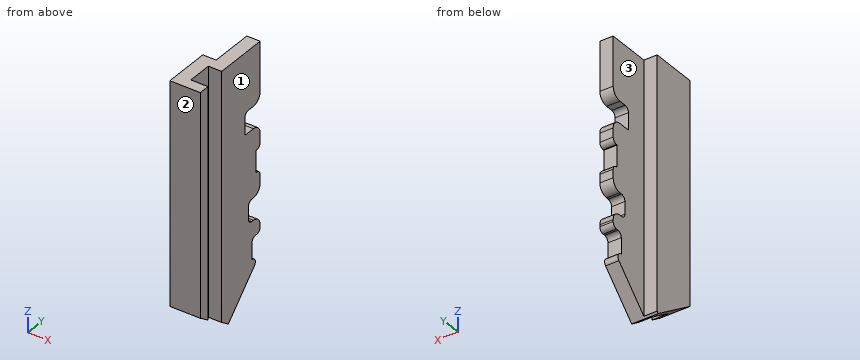
from build123d import *

# Parameters (mm, degrees)
BOSS_EXTRUDE1_DEPTH     = 13.28
CUT_EXTRUDE1_DEPTH      = 14.53406443
CUT_EXTRUDE1_DEPTH_BACK = 14.53406443
CUT_EXTRUDE5_DEPTH      = 0.29
CUT_EXTRUDE6_DEPTH      = 1.13
CUT_EXTRUDE7_DEPTH      = 0.87
CUT_EXTRUDE8_DEPTH      = 0.6
FILLET7_R               = 0.5
FILLET8_R               = 0.5
FILLET13_R              = 0.25
FILLET14_R              = 0.25
FILLET15_R              = 0.5
FILLET16_R              = 0.5
FILLET18_R              = 0.25
FILLET19_R              = 0.25
FILLET20_R              = 0.25
FILLET21_R              = 0.25
FILLET23_R              = 0.25
FILLET25_R              = 0.25


with BuildPart() as part:
    # Sketch1 → Boss-Extrude1 (new body)
    with BuildSketch(Plane.XY):
        Polygon((0, 0), (0, 2.28), (0.7, 2.28), (0.7, -0.58), (0, -0.58), (0, -1.88), (0.9, -1.88), (0.9, -2.45), (-0.7, -2.45), (-0.7, 0), align=None)
    extrude(amount=BOSS_EXTRUDE1_DEPTH)

    # Sketch2 → Cut-Extrude1 (cut, two sides: drawn at the far end of the back side and taken through both)
    with BuildSketch(Plane(origin=(0, 0, 0), x_dir=(0, 0, -1), z_dir=(1, 0, 0)).offset(-CUT_EXTRUDE1_DEPTH_BACK)):
        Polygon((0.8, -2.75), (0.8, -0.085), (0.8, 2.58), (-2.665, 2.58), (0, -0.085), (-1.866053089, -2.75), align=None)
    extrude(amount=CUT_EXTRUDE1_DEPTH + CUT_EXTRUDE1_DEPTH_BACK, mode=Mode.SUBTRACT)

    # 3DSketch1 → Cut-Extrude5 (cut)
    with BuildSketch(Plane(origin=(0.7, 2.28, 7.8225), x_dir=(-0.5199469468957453, 0, -0.8541985556144386), z_dir=(0, 1, 0))):
        Polygon((0, 0), (0.982328339, -0.597938989), (1.346291202, 0), (0.363962863, 0.597938989), align=None)
    extrude(amount=-CUT_EXTRUDE5_DEPTH, mode=Mode.SUBTRACT)

    # 3DSketch1<3> → Cut-Extrude6 (cut)
    with BuildSketch(Plane(origin=(0, 2.28, 10.196397445), x_dir=(0.5199469468957453, 0, -0.8541985556144386), z_dir=(0, 1, 0))):
        Polygon((0, 0), (0.982328339, 0.597938989), (1.346291202, 0), (0.363962863, -0.597938989), align=None)
    extrude(amount=-CUT_EXTRUDE6_DEPTH, mode=Mode.SUBTRACT)

    # 3DSketch1<4> → Cut-Extrude7 (cut)
    with BuildSketch(Plane(origin=(0, 2.28, 5.478611146), x_dir=(0.519345577670118, 0, -0.8545643164528294), z_dir=(0, 1, 0))):
        Polygon((0, 0), (0.984308217, 0.598195022), (1.347850122, 0), (0.363541904, -0.598195022), align=None)
    extrude(amount=-CUT_EXTRUDE7_DEPTH, mode=Mode.SUBTRACT)

    # 3DSketch1<5> → Cut-Extrude8 (cut)
    with BuildSketch(Plane(origin=(0, 2.28, 10.196397445), x_dir=(0.08902885316147792, 0, -0.9960290474201804), z_dir=(0, -1, 0))):
        Polygon((0, 0), (1.145433405, -0.102383181), (1.207753602, 0.594837152), (0.062320197, 0.697220333), align=None)
        Polygon((4.699052194, -0.420019104), (5.846302971, -0.522564728), (5.908623168, 0.174655605), (4.761372391, 0.277201229), align=None)
        Polygon((6.698507562, -0.598738006), (7.800299337, -0.697220333), (7.862619534, 0), (6.760827759, 0.098482327), align=None)
    extrude(amount=CUT_EXTRUDE8_DEPTH, mode=Mode.SUBTRACT)

    # Fillet7
    fillet7_edges = [part.edges().sort_by_distance(p)[0] for p in [
        (0.35, 2.28, 9.046397445),
    ]]
    fillet(fillet7_edges, radius=FILLET7_R)

    # Fillet8
    fillet8_edges = [part.edges().sort_by_distance(p)[0] for p in [
        (0.35, 2.28, 10.196397445),
    ]]
    fillet(fillet8_edges, radius=FILLET8_R)

    # Fillet13
    fillet13_edges = [part.edges().sort_by_distance(p)[0] for p in [
        (0.35, 2.28, 6.6725),
    ]]
    fillet(fillet13_edges, radius=FILLET13_R)

    # Fillet14
    fillet14_edges = [part.edges().sort_by_distance(p)[0] for p in [
        (0.35, 2.28, 7.8225),
    ]]
    fillet(fillet14_edges, radius=FILLET14_R)

    # Fillet15
    fillet15_edges = [part.edges().sort_by_distance(p)[0] for p in [
        (0.35, 2.28, 5.478611146),
    ]]
    fillet(fillet15_edges, radius=FILLET15_R)

    # Fillet16
    fillet16_edges = [part.edges().sort_by_distance(p)[0] for p in [
        (0.35, 2.28, 4.326786528),
    ]]
    fillet(fillet16_edges, radius=FILLET16_R)

    # Fillet18
    fillet18_edges = [part.edges().sort_by_distance(p)[0] for p in [
        (0.35, 2.28, 3.471184381),
    ]]
    fillet(fillet18_edges, radius=FILLET18_R)

    # Fillet19
    # the kernel refuses this fillet: 0.25 mm, written as the material it takes off along each edge
    with BuildSketch(Plane(origin=(2.208795436, 2.28, 2.365), x_dir=(0, -1, 0), z_dir=(-1, 0, 0))) as fillet19_piece_1:
        with BuildLine():
            CenterArc((0.603528489, -0.249975098), FILLET19_R, 90.808696936, 134.191303064)
            Line((0.426751794, -0.426751794), (0.42321626, -0.430287327))
            Line((0.42321626, -0.430287327), (-0.003535534, -0.003535534))
            Line((-0.003535534, -0.003535534), (0, 0.005))
            ThreePointArc((0, 0.005), (0.3, 0.005), (0.59992943, 0.004999502))
            Line((0.59992943, 0.004999502), (0.6, 0))
        make_face()
    extrude(amount=3.717590871, mode=Mode.SUBTRACT)

    # Fillet20
    fillet20_edges = [part.edges().sort_by_distance(p)[0] for p in [
        (0.35, 1.68, 3.471184381),
    ]]
    fillet(fillet20_edges, radius=FILLET20_R)

    # Fillet21
    fillet21_edges = [part.edges().sort_by_distance(p)[0] for p in [
        (0.35, 1.41, 4.326786528),
    ]]
    fillet(fillet21_edges, radius=FILLET21_R)

    # Fillet23
    fillet23_edges = [part.edges().sort_by_distance(p)[0] for p in [
        (0.35, 1.41, 5.478611146),
    ]]
    fillet(fillet23_edges, radius=FILLET23_R)

    # Fillet25
    fillet25_edges = [part.edges().sort_by_distance(p)[0] for p in [
        (0.35, 1.15, 10.196397445),
    ]]
    fillet(fillet25_edges, radius=FILLET25_R)


solid = part.part
Source: CAD feature listing. Evaluate the final solid. Frame: model axes, mm. Face numbers are marked on the shaded views. A direction names the side the tool comes from. Round coordinates to 2 decimals unless told otherwise and drop trailing zeros. Order: outer loops, then holes, each group sorted by start corner. A loop starts at its lowest first (then second) coordinate and runs counter-clockwise, first axis right, second up. Notation, with made-up numbers: (1, 42.5) - (38, 42.5) arc R27 cw to (38, 60.5) - close; hole circle Ø6 at (27, 76). An arc over 180 degrees is marked (long way). Use a Markdown table: item, result. Add a question column.
1. Set-up query: the marked faces 1, 2 and 3. Return all of +Z, -Z, +X, -X, +Y, -Y with unobstructed straight access to the full face (end or side cutting, diameter ignored); none if empty.
2. Section query B-B (x = -0.2). Return the cut outline in (y, z) (3 decimals), then the cut area to 3 significant figures.
3. Line query: probe 1 along Z at (x, y) = (0.45, 2.05); probe 2 along Y at (x, z) = (0.45, 11); probe 3 along X at (y, z) = (0.6, 6.75). Output: solid intervals per line, ascending.
4. First-contact query: pin 1 (0.7 mm diameter, centred on x = 0.5, z = 10, fed in from +Y); pin 2 (2.5 mm diameter, centred on y = 1, z = 6.5, fed in from -X); pin 3 (1 mm diameter, centred on y = -1, z = 6.5, fed in from +X); pin 4 (0.8 mm diameter, centred on x = 0.5, z = 9.5, fed in from +Y). Flat tips, straight axial feed; report the tip coordinate or a pass-through.
5. Section query A-A (z = 11). Return the cut outline in (x, y), then the cut area to 3 significant figures.
6. Section query C-C (z = 7.5). Return the cut outline in (x, y).
7. Section query D-D (y = 0.4). Return the cut outline in (x, z) (3 decimals), then the cut area to 3 significant figures.
Derived:
| question | item | result |
|---|---|---|
| 1 | face 1 | +Z, -Z, +X, +Y |
| 1 | face 2 | +Z, -Z, +X, -X, -Y |
| 1 | face 3 | +Z, -Z, -X, +Y |
| 2 | outline | (-2.45, 1.656) - (-0.085, 0) - (0, 0.085) - (0, 13.28) - (-2.45, 13.28) - close |
| 2 | area | 30.6 mm2 |
| 3 | probe 1 | 3.47 to 4.25, 5.56 to 6.67, 7.82 to 8.97, 10.28 to 13.28 |
| 3 | probe 2 | -2.45 to -1.88, -0.58 to 2.28 |
| 3 | probe 3 | 0 to 0.7 |
| 4 | pin 1 | y = 2.14 |
| 4 | pin 2 | x = -0.7 |
| 4 | pin 3 | x = 0.7 |
| 4 | pin 4 | y = 1.15 |
| 5 | outline | (-0.7, -2.45) - (0.9, -2.45) - (0.9, -1.88) - (0, -1.88) - (0, -0.58) - (0.7, -0.58) - (0.7, 2.28) - (0, 2.28) - (0, 0) - (-0.7, 0) - close |
| 5 | area | 4.23 mm2 |
| 6 | outline | (-0.7, -2.45) - (0.9, -2.45) - (0.9, -1.88) - (0, -1.88) - (0, -0.58) - (0.7, -0.58) - (0.7, 1.99) - (0, 1.99) - (0, 0) - (-0.7, 0) - close |
| 7 | outline | (0, 0.485) - (0.7, 0.485) - (0.7, 13.28) - (0, 13.28) - close |
| 7 | area | 8.96 mm2 |
